```python
from build123d import *


with BuildPart() as part:
    # Sketch1 → Revolve1 (revolve)
    with BuildSketch(Plane(origin=(0, 0, 0), x_dir=(0, 0, -1), z_dir=(1, 0, 0)), mode=Mode.PRIVATE) as revolve1_sk:
        with BuildLine():
            Line((-7.46, 0), (-28.415, 0))
            Line((-28.415, 0), (-28.415, 3))
            ThreePointArc((-28.415, 3), (-27.829213562, 4.414213562), (-26.415, 5))
            Line((-26.415, 5), (-10.05, 5))
            Line((-10.05, 5), (-10.05, 7.5))
            Line((-10.05, 7.5), (-8.5, 7.5))
            Line((-8.5, 7.5), (-8.4, 16.8))
            Line((-8.4, 16.8), (-7.46, 16.8))
            Line((-7.46, 16.8), (-7.46, 0))
        make_face()
    revolve(revolve1_sk.sketch.rotate(Axis((0, 0, 0), (0, 1, 0)), 180), axis=Axis((0, 0, 0), (0, 1, 0)))


solid = part.part
```
Can you work these out from the model? Positions are in its coordinate system, mm. A direction names the side the tool comes from. Give positions to 0.01 mm unless a question says otherwise; leave off trailing zeros. Loops run counter-clockwise (first coordinate to the right, second up) from the corner with the lowest first, then second, coordinate; pieces in that order, holes last. Notation, with made-up numbers: M 81,-10 L 111,-10 A8 cw 111,-5 Z; hole C 64.5,-11 d6. An arc over 180 degrees is marked long. One line per question, with ' | ' between items. Start each with the question number.
Q1. For faces 1 (the conical face through (-2.54, 12.22, -8.06)), 2 (the cylindrical face through (-8.54, 1.52, -27.1)), which set-ups out of +Z, -Z, +X, -X, +Y, -Y let a thin tool reach every point of the face, with its end or its side?
Q2. If we section it at A-A (y = 1): Please give me the cut outline in (x, z) (3 decimals), plus the area to 3 significant figures.
Q3. If I drill on line 1 (Y direction, x = -1, z = 25); line 2 (X direction, y = 11.5, z = 0); line 3 (Y direction, x = 8.5, z = 26), over which ranges is the centre line in solid material (lowest first)? Write a range as from..to.
Q4. For pin 1 Ø5 at (y, z) = (9.5, -16.5) entering from +X; pin 2 Ø5 at (x, z) = (-11, -7) entering from +Y; pin 3 Ø8 at (x, y) = (5.5, 13) entering from -Z; pin 4 Ø2 at (y, z) = (2, -11) entering from -X, each with a flat end and sliding along its axis, tell me the tip position at first contact or that it passes through.
Q5. If we mould it in two halves opening along Z, with no side actions, what happens to faces 3 (the cylindrical face through (-0.44, 6.27, 10.04)), 4 (the flat face through (-4.5, 7.5, 7.5)), 5 (the cylindrical face through (-7.397, 8.282, 0.971))? For each: +Z half, -Z half, draft (parallel to the pull), parting line (faces both ways), or undercut.
Computed:
1) face 1: +Y | face 2: +Y, -Y
2) outline: C 0,0 d56.83; hole C 0,0 d14.92 | area: 2,360 mm²
3) line 1: y = 0..5 | line 2: x = -8.46..-7.46, 7.46..8.46 | line 3: y = 0..4.77
4) pin 1: passes through | pin 2: stops at y = 5 | pin 3: stops at z = -8.31 | pin 4: stops at x = -26.6
5) face 3: parting line | face 4: draft | face 5: undercut
